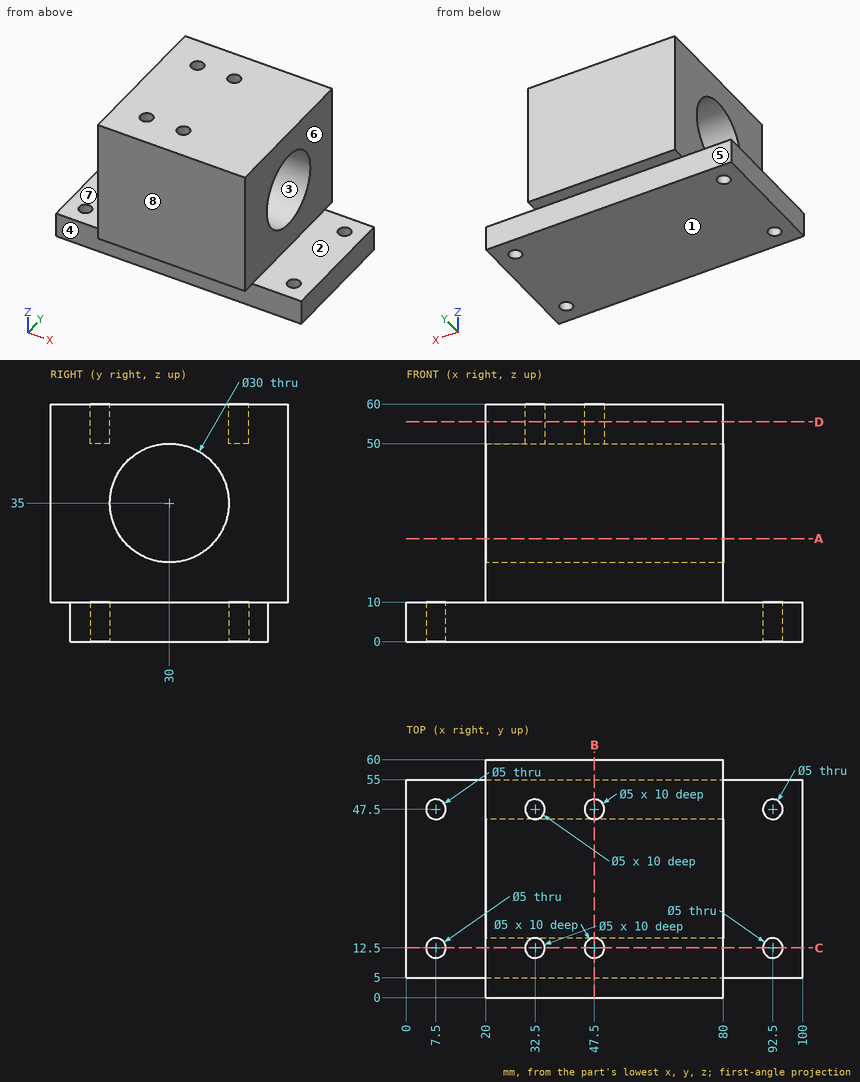
Geometry: see drawing. Coordinates: mm, zero at the bounding-box minimum. A direction names the side the tool comes from. Give positions to 0.01 mm unless a question says otherwise; leave off trailing zeros. Loops run counter-clockwise (first coordinate to the right, second up) from the corner with the lowest first, then second, coordinate; pieces in that order, holes last. Notation, with made-up numbers: (11.5, 68.25) -> (26.5, 68.25) arc R10 cw to (26.5, 77.25) -> close; hole circle Ø7 at (79, -18.75). An arc over 180 degrees is marked (long way). Answer as a JSON object with one key per item and string values. Group by question number.
Item 1: Pin query (flat end, axial travel): P1, Ø1, axis at x = 70, z = 7.5, coming from the +Y side; P2, Ø10, axis at y = 36, z = 34, coming from the -X side; P3, Ø3, axis at y = 52, z = 46, coming from the +X side; P4, Ø4, axis at x = 47.5, y = 12.5, coming from the +Z side. Return the tip coordinate at first contact, or that it passes through.
Item 2: Pull-direction query (Z, two-part tool) for the marked faces 1, 2, 3 and 4; classes: released by +Z, released by -Z, zero draft, split by the parting line, or undercut.
Item 3: Line query: probe 1 along Y at (x, z) = (32.5, 58); probe 2 along Y at (x, z) = (38.5, 35); probe 3 along Y at (x, z) = (7.5, 5.25). Output: solid intervals per line, ascending.
Item 4: Cut plane A-A, the plane z = 26. Return the cut outline in (x, y).
Item 5: Reachability of the marked faces 5, 6, 7 and 8 from +Z, -Z, +X, -X, +Y, -Y: full face, straight path, thin tool, end or side. Return the list, or none.
Item 6: Cut plane B-B, the plane x = 47.5. Return the cut outline in (y, z).
Item 7: Cut plane C-C, the plane y = 12.5. Return the cut outline in (x, z), and give its area (3 significant figures).
Item 8: Cut plane D-D, the plane z = 55.5. Return the cut outline in (x, y), and give its area (3 significant figures).
Checks:
{
 "1": {"P1": "stops at y = 55", "P2": "passes through", "P3": "stops at x = 80", "P4": "stops at z = 50"},
 "2": {"face 1": "released by -Z", "face 2": "released by +Z", "face 3": "undercut", "face 4": "zero draft"},
 "3": {"probe 1": "y = 0 to 10, 15 to 45, 50 to 60", "probe 2": "y = 0 to 15, 45 to 60", "probe 3": "y = 5 to 10, 15 to 45, 50 to 55"},
 "4": {"outline": "(20, 0) -> (80, 0) -> (80, 18) -> (20, 18) -> close; (20, 42) -> (80, 42) -> (80, 60) -> (20, 60) -> close"},
 "5": {"face 5": "-Z, +X, -X, +Y", "face 6": "+Z, +X, +Y, -Y", "face 7": "+Z, -X, +Y, -Y", "face 8": "+Z, -Z, +X, -X, -Y"},
 "6": {"outline": "(0, 10) -> (5, 10) -> (5, 0) -> (55, 0) -> (55, 10) -> (60, 10) -> (60, 60) -> (50, 60) -> (50, 50) -> (45, 50) -> (45, 60) -> (15, 60) -> (15, 50) -> (10, 50) -> (10, 60) -> (0, 60) -> close; hole circle Ø30 at (30, 35)"},
 "7": {"outline": "(0, 0) -> (5, 0) -> (5, 10) -> (0, 10) -> close; (10, 0) -> (90, 0) -> (90, 10) -> (80, 10) -> (80, 60) -> (50, 60) -> (50, 50) -> (45, 50) -> (45, 60) -> (35, 60) -> (35, 50) -> (30, 50) -> (30, 60) -> (20, 60) -> (20, 10) -> (10, 10) -> close; (95, 0) -> (100, 0) -> (100, 10) -> (95, 10) -> close", "area": "3,800 mm²"},
 "8": {"outline": "(20, 0) -> (80, 0) -> (80, 60) -> (20, 60) -> close; hole circle Ø5 at (32.5, 12.5); hole circle Ø5 at (32.5, 47.5); hole circle Ø5 at (47.5, 12.5); hole circle Ø5 at (47.5, 47.5)", "area": "3,520 mm²"}
}
